For this review, take the finished solid that the model builds, in its own axes (mm). Face numbers are marked on the shaded views. A direction names the side the tool comes from. Give positions to 0.01 mm unless a question says otherwise; leave off trailing zeros. Loops run counter-clockwise (first coordinate to the right, second up) from the corner with the lowest first, then second, coordinate; pieces in that order, holes last. Notation, with made-up numbers: (52, 69.5) -> (79, 69.5) arc R33 ccw to (79, 106.5) -> close; hole circle Ø4 at (43, -6.75). An arc over 180 degrees is marked (long way). Answer as CSV lines item,"result". Start each with the question number.
Item 1: Add section A-A on z = -65. State the section outline as (x, y) points.
Item 2: Machinability: for the marked faces 1 and 2, which of the approach directions +Z, -Z, +X, -X, +Y, -Y give a long, thin tool a straight path to every point of the face, cutting with its end or side? Answer none if there is none.
Item 3: For L1, parallel to Z at x = 35.5, y = 359.5; L2, parallel to Y at x = 32, z = -142.5, list the stretches that pass through material, from the lowest coordinate up. Write a range as from..to.
Item 4: Clearance check with flat-ended pins moving along their axes: P1, Ø12, axis at x = 12, y = 200, coming from the -Z side; P2, Ø2, axis at x = 9, z = -45.5, coming from the +Y side. State where each tip first meets the part, or that it passes through.
Item 5: Add section C-C on x = 20. State how many separate pieces and enclosed holes the cut face has, plus the area to 3 significant figures.
Item 6: Add section B-B on y = 250. State the section outline as (x, z) points.
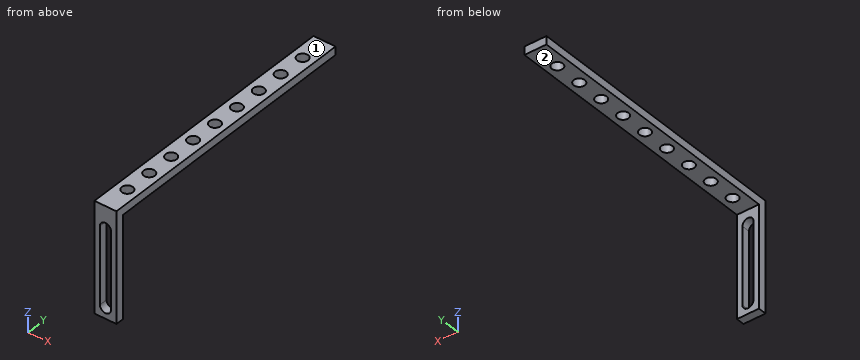
```python
from build123d import *

# Parameters (mm, degrees)
EXTRUDE_1_DEPTH     = 40
SKETCH_2_R          = 10.05
CUT_EXTRUDE_1_DEPTH = 201
CUT_EXTRUDE_2_REACH = 502


with BuildPart() as part:
    # Эскиз1 → Бобышка-Вытянуть1 (new body)
    with BuildSketch(Plane(origin=(0, 0, 0), x_dir=(0, 0, -1), z_dir=(1, 0, 0))):
        Polygon((0, 0), (0, 500), (15, 500), (15, 15), (200, 15), (200, 0), align=None)
    extrude(amount=EXTRUDE_1_DEPTH)

    # Эскиз2 → Вырез-Вытянуть1 (cut, through all)
    with BuildSketch(Plane.XY):
        with Locations((20, 50)):
            Circle(SKETCH_2_R)
        with Locations((20, 100)):
            Circle(SKETCH_2_R)
        with Locations((20, 150)):
            Circle(SKETCH_2_R)
        with Locations((20, 200)):
            Circle(SKETCH_2_R)
        with Locations((20, 250)):
            Circle(SKETCH_2_R)
        with Locations((20, 300)):
            Circle(SKETCH_2_R)
        with Locations((20, 350)):
            Circle(SKETCH_2_R)
        with Locations((20, 400)):
            Circle(SKETCH_2_R)
        with Locations((20, 450)):
            Circle(SKETCH_2_R)
    extrude(amount=-CUT_EXTRUDE_1_DEPTH, mode=Mode.SUBTRACT)

    # Эскиз3 → Вырез-Вытянуть2 (cut, up to next)
    with BuildSketch(Plane.XZ, mode=Mode.PRIVATE) as cut_extrude_2_sk1:
        with BuildLine():
            Line((9.95, -40), (9.95, -180))
            ThreePointArc((9.95, -180), (20, -190.05), (30.05, -180))
            Line((30.05, -180), (30.05, -40))
            ThreePointArc((30.05, -40), (20, -29.95), (9.95, -40))
        make_face()
    cut_extrude_2_tool1 = extrude(cut_extrude_2_sk1.sketch, amount=-CUT_EXTRUDE_2_REACH, mode=Mode.PRIVATE) & part.part
    add(cut_extrude_2_tool1.solids().sort_by_distance((20, 0, -110))[0], mode=Mode.SUBTRACT)


solid = part.part
```
Computed values:
1,outline,"(0, 0) -> (9.95, 0) -> (9.95, 15) -> (0, 15) -> close; (30.05, 0) -> (40, 0) -> (40, 15) -> (30.05, 15) -> close"
2,face 1,"+Z, +X, -X, +Y, -Y"
2,face 2,"-Z, +X, -X, +Y"
3,L1,"-15..0"
3,L2,"0..15"
4,P1,"z = -15"
4,P2,"y = 15"
5,separate pieces,"11"
5,enclosed holes,"0"
5,area,"5,160 mm²"
6,outline,"(0, -15) -> (9.95, -15) -> (9.95, 0) -> (0, 0) -> close; (30.05, -15) -> (40, -15) -> (40, 0) -> (30.05, 0) -> close"
